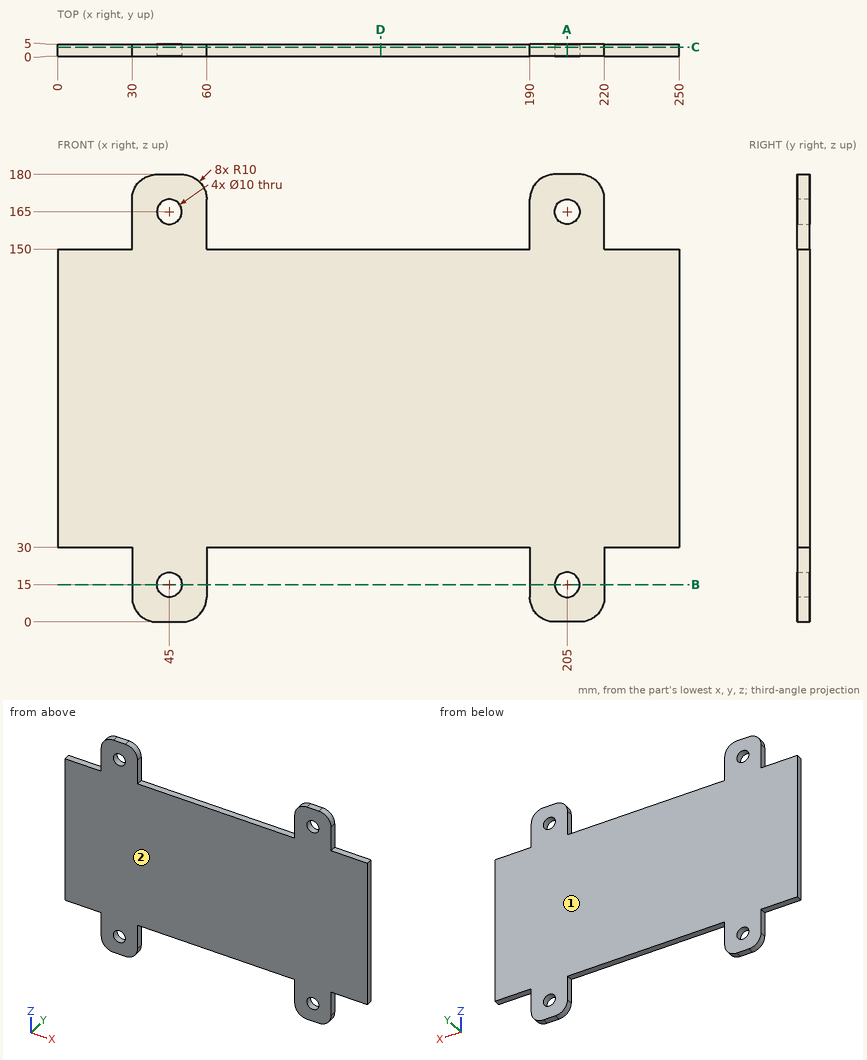
Part print with two shaded views. Sizes in mm from the minimum x, y, z corner. Round coordinates to 2 decimals unless told otherwise and drop trailing zeros. Loops run counter-clockwise (first coordinate to the right, second up) from the corner with the lowest first, then second, coordinate; pieces in that order, holes last. Notation, with made-up numbers: M 59.5,34.5 L 84.5,34.5 A24 cw 84.5,58.5 Z; hole C -22,80.5 d9. An arc over 180 degrees is marked long. Return JSON: item names as keys, results as strings. Group by question number.
(1) Drop flat-ended pins along their axis: P1, Ø2.5, axis at y = 2.5, z = 160, coming from the +X side; P2, Ø2, axis at x = 90.5, y = 4, coming from the -Z side; P3, Ø3, axis at y = 2, z = 62.5, coming from the -X side; P4, Ø1.5, axis at x = 100.5, y = 3, coming from the +Z side. Give the stop position or say it passes through.
(2) Wall check: probe 1 along X at (y, z) = (3.5, 15); probe 2 along Z at (x, y) = (205, 1.7); probe 3 along Z at (x, y) = (227.5, 3.95). Give the ranges that are in metal, low to high. Write a range as [from, to].
(3) Saw through at C-C, the plane y = 3.75. Give the number of separate pieces and of enclosed holes in the cut face, and give its area (3 significant figures).
(4) Saw through at A-A, the plane x = 205. List the corners of the cut face in (y, z), and give its area (3 significant figures).
(5) Saw through at D-D, the plane x = 130. List the corners of the cut face in (y, z), and give its area (3 significant figures).
(6) Mould opens along Y. For the marked faces 1 and 2 say: +Y half, -Y half, draft (parallel to the pull), parting line (faces both ways), or undercut.
(7) Saw through at B-B, the plane z = 15. List the corners of the cut face in (x, y), and give its area (3 significant figures).
Answer list:
{
 "1": {"P1": "x = 220", "P2": "z = 30", "P3": "x = 0", "P4": "z = 150"},
 "2": {"probe 1": "[30, 40], [50, 60], [190, 200], [210, 220]", "probe 2": "[0, 10], [20, 160], [170, 180]", "probe 3": "[30, 150]"},
 "3": {"separate pieces": "1", "enclosed holes": "4", "area": "33,100 mm2"},
 "4": {"outline": "M 0,0 L 5,0 L 5,10 L 0,10 Z; M 0,20 L 5,20 L 5,160 L 0,160 Z; M 0,170 L 5,170 L 5,180 L 0,180 Z", "area": "800 mm2"},
 "5": {"outline": "M 0,30 L 5,30 L 5,150 L 0,150 Z", "area": "600 mm2"},
 "6": {"face 1": "+Y half", "face 2": "-Y half"},
 "7": {"outline": "M 30,0 L 40,0 L 40,5 L 30,5 Z; M 50,0 L 60,0 L 60,5 L 50,5 Z; M 190,0 L 200,0 L 200,5 L 190,5 Z; M 210,0 L 220,0 L 220,5 L 210,5 Z", "area": "200 mm2"}
}
